Source: CAD feature listing. Evaluate the final solid. Frame: model axes, mm. Face numbers are marked on the shaded views. Give positions to 0.01 mm unless a question says otherwise; leave off trailing zeros. Write each loop counter-clockwise with the first axis right and the second up, starting at its lowest first coordinate (ties: lowest second). Pieces come first, ordered by that corner, then holes. Notation, with made-up numbers: M 32,73 L 41,73 A6 ccw 41,83 Z; hole C 24,-38 d10. An arc over 180 degrees is marked long. Return JSON: item names as keys, results as strings.
```python
from build123d import *

# Parameters (mm, degrees)
SKETCH_R              = 16.8
PAD_DEPTH             = 18.2
SKETCH001_R           = 1.25
POCKET_DEPTH          = 2
POLARPATTERN_COUNT    = 4
SKETCH002_R           = 4.15
POCKET001_DEPTH       = 18.201
SKETCH003_R           = 1.25
POCKET002_DEPTH       = 3
POLARPATTERN001_COUNT = 4
SKETCH004_R           = 6
SKETCH004_R_2         = 4.15
PAD001_DEPTH          = 1.8
SKETCH005_R           = 16.8
SKETCH005_R_2         = 15.4
POCKET003_DEPTH       = 1.3
SKETCH006_W           = 11.8
SKETCH006_H           = 0.3
CHAMFER_SIZE          = 2
CHAMFER001_SIZE       = 0.1
CHAMFER002_SIZE       = 0.1
CHAMFER003_SIZE       = 0.1
CHAMFER004_SIZE       = 0.1
CHAMFER005_SIZE       = 0.1
POCKET004_DEPTH       = 3


with BuildPart() as part:
    # Sketch → Pad (new body)
    with BuildSketch(Plane.XY):
        Circle(SKETCH_R)
    extrude(amount=PAD_DEPTH)

    # Sketch001 (on Face3 of Pad) → Pocket (cut)
    with BuildSketch(Plane.XY.offset(18.2)):
        with Locations((0, 8.25)):
            Circle(SKETCH001_R)
    pocket = extrude(amount=-POCKET_DEPTH, mode=Mode.SUBTRACT)

    # PolarPattern: Pocket ×4 about axis
    polarpattern_axis = Axis((0, 0, 18.2), (0, 0, 1))
    for i in range(1, POLARPATTERN_COUNT):
        add(pocket.rotate(polarpattern_axis, i * 360 / POLARPATTERN_COUNT), mode=Mode.SUBTRACT)

    # Sketch002 (on Face3 of PolarPattern) → Pocket001 (cut, through all)
    with BuildSketch(Plane.XY.offset(18.2)):
        Circle(SKETCH002_R)
    extrude(amount=-POCKET001_DEPTH, mode=Mode.SUBTRACT)

    # Sketch003 (on Face2 of Pocket001) → Pocket002 (cut)
    with BuildSketch(Plane(origin=(0, 0, 0), x_dir=(1, 0, 0), z_dir=(0, 0, -1))):
        with Locations((0, 11.25)):
            Circle(SKETCH003_R)
    pocket002 = extrude(amount=-POCKET002_DEPTH, mode=Mode.SUBTRACT)

    # PolarPattern001: Pocket002 ×4 about axis
    polarpattern001_axis = Axis((0, 0, 0), (0, 0, -1))
    for i in range(1, POLARPATTERN001_COUNT):
        add(pocket002.rotate(polarpattern001_axis, i * 360 / POLARPATTERN001_COUNT), mode=Mode.SUBTRACT)

    # Sketch004 (on Face2 of PolarPattern001) → Pad001 (join)
    with BuildSketch(Plane(origin=(0, 0, 0), x_dir=(1, 0, 0), z_dir=(0, 0, -1))):
        Circle(SKETCH004_R)
        Circle(SKETCH004_R_2, mode=Mode.SUBTRACT)
    extrude(amount=PAD001_DEPTH)

    # Sketch005 (on Face2 of Pad001) → Pocket003 (cut)
    with BuildSketch(Plane(origin=(0, 0, 0), x_dir=(1, 0, 0), z_dir=(0, 0, -1))):
        Circle(SKETCH005_R)
        Circle(SKETCH005_R_2, mode=Mode.SUBTRACT)
    extrude(amount=-POCKET003_DEPTH, mode=Mode.SUBTRACT)

    # Sketch006 → Groove (revolve, cut)
    with BuildSketch(Plane.XZ):
        with Locations((-10.9, 5.15)):
            Rectangle(SKETCH006_W, SKETCH006_H)
    revolve(axis=Axis((0, 0, 0), (0, 0, 1)), mode=Mode.SUBTRACT)

    # Chamfer
    chamfer_edges = [part.edges().sort_by_distance(p)[0] for p in [
        (-16.8, 0, 18.2),
    ]]
    chamfer(chamfer_edges, length=CHAMFER_SIZE)

    # Chamfer001
    chamfer001_edges = [part.edges().sort_by_distance(p)[0] for p in [
        (-16.8, 0, 1.3),
    ]]
    chamfer(chamfer001_edges, length=CHAMFER001_SIZE)

    # Chamfer002
    chamfer002_edges = [part.edges().sort_by_distance(p)[0] for p in [
        (-15.4, 0, 0),
    ]]
    chamfer(chamfer002_edges, length=CHAMFER002_SIZE)

    # Chamfer003
    chamfer003_edges = [part.edges().sort_by_distance(p)[0] for p in [
        (-15.4, 0, 1.3),
    ]]
    chamfer(chamfer003_edges, length=CHAMFER003_SIZE)

    # Chamfer004
    chamfer004_edges = [part.edges().sort_by_distance(p)[0] for p in [
        (0, -16.8, 5),
    ]]
    chamfer(chamfer004_edges, length=CHAMFER004_SIZE)

    # Chamfer005
    chamfer005_edges = [part.edges().sort_by_distance(p)[0] for p in [
        (5, 0, 5.3),
        (0, 16.8, 5.3),
        (0, -16.8, 5.3),
    ]]
    chamfer(chamfer005_edges, length=CHAMFER005_SIZE)

    # Sketch007 (on Face29 of Chamfer005) → Pocket004 (cut)
    with BuildSketch(Plane(origin=(0, 0, 0), x_dir=(1, 0, 0), z_dir=(0, 0, -1))):
        with BuildLine():
            ThreePointArc((7.884241, 9.298454), (6.82358, 9.298454), (6.82358, 8.237794))
            Line((6.82358, 8.237794), (8.237794, 6.82358))
            ThreePointArc((8.237794, 6.82358), (9.298454, 6.82358), (9.298454, 7.884241))
            Line((9.298454, 7.884241), (7.884241, 9.298454))
        make_face()
    extrude(amount=-POCKET004_DEPTH, mode=Mode.SUBTRACT)


solid = part.part
```
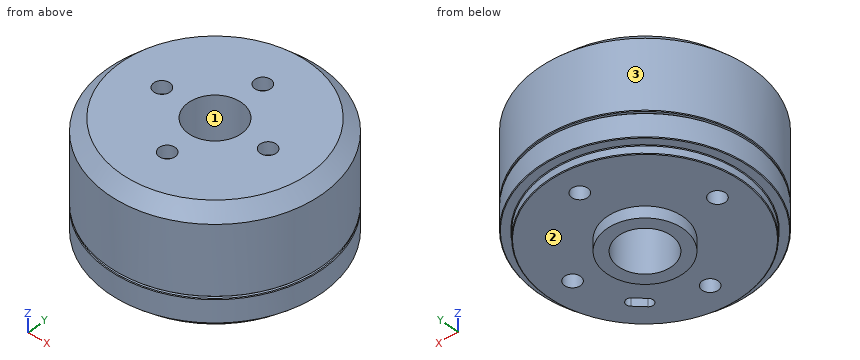
1) Draft query along X for the marked faces 1, 2 and 3. Return one class per face: released by +X, released by -X, zero draft, split by the parting line, or undercut.
Numbers:
{"face 1": "undercut", "face 2": "zero draft", "face 3": "split by the parting line"}
2) Cut plane A-A, the plane z = 15.5. Return the cut outline in (x, y), then the cut area to 3 significant figures.
Numbers:
{"outline": "C 0,0 d33.6; hole C 0,0 d8.3", "area": "833 mm²"}
3) Contact query for flat-ended pins moving along their axis: pin 1 Ø3 at (x, y) = (-8.25, 0) entering from -Z; pin 2 Ø10 at (x, y) = (-4, -8) entering from -Z; pin 3 Ø2 at (y, z) = (10.5, 13.5) entering from +X; pin 4 Ø0.8 at (x, y) = (0.5, 11) entering from -Z. Output: stop coordinate, or through.
Numbers:
{"pin 1": "stops at z = 0", "pin 2": "stops at z = -1.8", "pin 3": "stops at x = 13.86", "pin 4": "stops at z = 3"}
4) Line query: line 1 (Z direction, x = 12, y = -5.5); line 2 (X direction, y = -0.5, z = 1); line 3 (Y direction, x = 0, z = 0.9). Output: solid intervals per line, ascending. Write a range as [from, to].
Numbers:
{"line 1": "z = [0, 5], [5.3, 18.2]", "line 2": "x = [-15.39, -12.4], [-10.1, -4.12], [4.12, 10.1], [12.4, 15.39]", "line 3": "y = [-15.4, -12.5], [-10, -4.15], [4.15, 10], [12.5, 15.4]"}
